```python
from build123d import *

# Parameters (mm, degrees)
SKETCH1_W               = 1500
SKETCH1_H               = 1600
SKETCH1_R               = 65
BOSS_EXTRUDE1_DEPTH     = 200
CUT_EXTRUDE1_DEPTH      = 1
CUT_EXTRUDE1_DEPTH_BACK = 1601


with BuildPart() as part:
    # Sketch1 → Boss-Extrude1 (new body)
    with BuildSketch(Plane(origin=(0, 0, 0), x_dir=(1, 0, 0), z_dir=(0, 1, 0))):
        with Locations((-48.109243697, 800)):
            Rectangle(SKETCH1_W, SKETCH1_H)
        with Locations((436.890756303, 1455)):
            Circle(SKETCH1_R, mode=Mode.SUBTRACT)
        with Locations((-48.109243697, 1455)):
            Circle(SKETCH1_R, mode=Mode.SUBTRACT)
        with Locations((-533.109243697, 1455)):
            Circle(SKETCH1_R, mode=Mode.SUBTRACT)
        with Locations((436.890756303, 145)):
            Circle(SKETCH1_R, mode=Mode.SUBTRACT)
        with Locations((-48.109243697, 145)):
            Circle(SKETCH1_R, mode=Mode.SUBTRACT)
        with Locations((-533.109243697, 145)):
            Circle(SKETCH1_R, mode=Mode.SUBTRACT)
    extrude(amount=BOSS_EXTRUDE1_DEPTH)

    # Sketch3 → Cut-Extrude1 (cut, two sides)
    with BuildSketch(Plane.XY) as cut_extrude1_sk:
        Polygon((-690.966386555, 200), (-754.956850499, 200), (-744.537815126, 167.358848998), (-701.385421928, 167.358848998), align=None)
        Polygon((676.176470588, 200), (612.186006644, 200), (622.605042017, 167.358848998), (665.757435215, 167.358848998), align=None)
        Polygon((569.033613445, 200), (505.043149501, 200), (515.462184874, 167.358848998), (558.614578072, 167.358848998), align=None)
        Polygon((466.176470588, 200), (402.186006644, 200), (412.605042017, 167.358848998), (455.757435215, 167.358848998), align=None)
        Polygon((359.033613445, 200), (295.043149501, 200), (305.462184874, 167.358848998), (348.614578072, 167.358848998), align=None)
        Polygon((256.176470588, 200), (192.186006644, 200), (202.605042017, 167.358848998), (245.757435215, 167.358848998), align=None)
        Polygon((149.033613445, 200), (85.043149501, 200), (95.462184874, 167.358848998), (138.614578072, 167.358848998), align=None)
        Polygon((46.176470588, 200), (-17.813993356, 200), (-7.394957983, 167.358848998), (35.757435215, 167.358848998), align=None)
        Polygon((-60.966386555, 200), (-124.956850499, 200), (-114.537815126, 167.358848998), (-71.385421928, 167.358848998), align=None)
        Polygon((-163.823529412, 200), (-227.813993356, 200), (-217.394957983, 167.358848998), (-174.242564785, 167.358848998), align=None)
        Polygon((-270.966386555, 200), (-334.956850499, 200), (-324.537815126, 167.358848998), (-281.385421928, 167.358848998), align=None)
        Polygon((-373.823529412, 200), (-437.813993356, 200), (-427.394957983, 167.358848998), (-384.242564785, 167.358848998), align=None)
        Polygon((-480.966386555, 200), (-544.956850499, 200), (-534.537815126, 167.358848998), (-491.385421928, 167.358848998), align=None)
        Polygon((-583.823529412, 200), (-647.813993356, 200), (-637.394957983, 167.358848998), (-594.242564785, 167.358848998), align=None)
    extrude(amount=CUT_EXTRUDE1_DEPTH, mode=Mode.SUBTRACT)
    extrude(cut_extrude1_sk.sketch, amount=-CUT_EXTRUDE1_DEPTH_BACK, mode=Mode.SUBTRACT)


solid = part.part
```
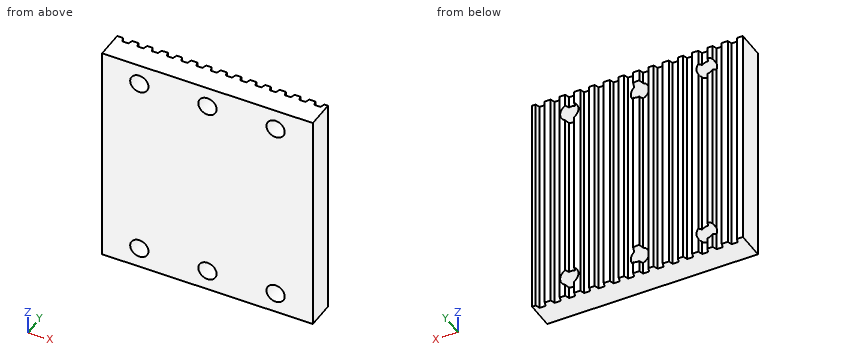
Build history of the part. All positions in model axes, mm. Round coordinates to 2 decimals unless told otherwise and drop trailing zeros. Order: outer loops, then holes, each group sorted by start corner. A loop starts at its lowest first (then second) coordinate and runs counter-clockwise, first axis right, second up. Notation, with made-up numbers: (9.25, 82.25) -> (51.25, 82.25) arc R13 ccw to (51.25, 96.25) -> close; hole circle Ø5 at (82, -33). An arc over 180 degrees is marked (long way). Answer in a Markdown table with one row per item.
1) Pin check, flat tip, straight feed: P1, Ø21.5, axis at x = -300, z = -731, coming from the +Y side. Stop position of the tip, or through.
Values:
| item | result |
|---|---|
| P1 | y = 167.36 |
2) Band-saw the part on A-A on y = 72.5. Give the cut face in (x, z).
Values:
| item | result |
|---|---|
| outline | (-798.11, -1600) -> (701.89, -1600) -> (701.89, 0) -> (-798.11, 0) -> close; hole circle Ø130 at (-533.11, -1455); hole circle Ø130 at (-533.11, -145); hole circle Ø130 at (-48.11, -1455); hole circle Ø130 at (-48.11, -145); hole circle Ø130 at (436.89, -1455); hole circle Ø130 at (436.89, -145) |
3) Band-saw the part on B-B on z = -145. Give the number of separate pieces and of enclosed holes in the cut face, and give its area (3 significant figures).
Values:
| item | result |
|---|---|
| separate pieces | 4 |
| enclosed holes | 0 |
| area | 204,000 mm2 |
4) Wall check: L1, parallel to X at y = 57.5, z = -145; L2, parallel to Z at x = -544.5, y = 157; L3, parallel to Z at x = 379.5, y = 101.5. Give the ranges that are in metal, low to high.
Values:
| item | result |
|---|---|
| L1 | -798.11 to -598.11, -468.11 to -113.11, 16.89 to 371.89, 501.89 to 701.89 |
| L2 | -1600 to -1518.99, -1391.01 to -208.99, -81.01 to 0 |
| L3 | -1600 to -1485.52, -1424.48 to -175.52, -114.48 to 0 |
